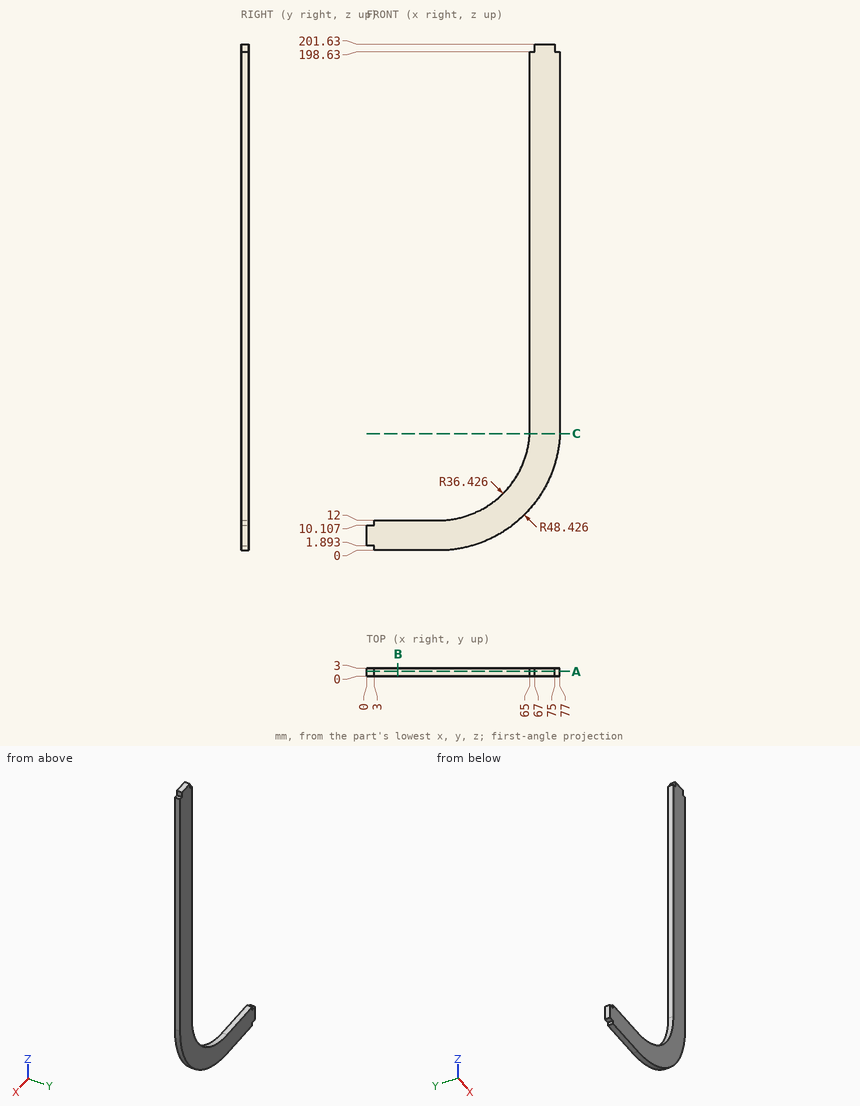
Here's the drawing with two shaded views (mm, measured from the low corner). I have some questions. Give positions to 0.01 mm unless a question says otherwise; leave off trailing zeros. Order: outer loops, then holes, each group sorted by start corner. A loop starts at its lowest first (then second) coordinate and runs counter-clockwise, first axis right, second up.
Q1. If I drill on line 1 along X through (y, z) = (0.85, 132); line 2 along Z through (x, y) = (18, 1.25); line 3 along Z through (x, y) = (47, 1.4) (1 decimal), over which ranges is the centre line in solid material (lowest first)?
Q2. Suppose I cut it at C-C, the plane z = 46.5. Write out the boundary of the cut face in (x, y).
Q3. I'm going to push flat-ended pins straight in: P1, Ø1.5, axis at y = 2, z = 199.5, coming from the -X side; P2, Ø1.5, axis at x = 45, y = 2, coming from the +Z side (1 decimal); P3, Ø0.6, axis at y = 1.5, z = 11, coming from the -X side. Where does each tip first touch, or does it pass through?
Q4. Suppose I cut it at A-A, the plane y = 1.8. Write out the boundary of the cut face in (x, z).
Q5. Suppose I cut it at B-B, the plane x = 12.5. Write out the boundary of the cut face in (y, z), and give its area (3 significant figures).
Solution:
1. line 1: x = 65 to 77
1. line 2: z = 0 to 12
1. line 3: z = 3.6 to 17
2. outline: (64.95, 0) - (76.96, 0) - (76.96, 3) - (64.95, 3) - close
3. P1: stops at x = 67
3. P2: stops at z = 16.3
3. P3: stops at x = 3
4. outline: (0, 1.89) - (3, 1.89) - (3, 0) - (28.57, 0) arc R48.43 ccw to (77, 48.43) - (77, 198.63) - (75, 198.63) - (75, 201.63) - (67, 201.63) - (67, 198.63) - (65, 198.63) - (65, 48.43) arc R36.43 cw to (28.57, 12) - (3, 12) - (3, 10.11) - (0, 10.11) - close
5. outline: (0, 0) - (3, 0) - (3, 12) - (0, 12) - close
5. area: 36.0 mm2
